```python
from build123d import *

# Parameters (mm, degrees)
SKETCH_1_R          = 3
EXTRUDE_1_DEPTH     = 8
SKETCH_2_R          = 1.5
CUT_EXTRUDE_1_DEPTH = 8
SKETCH_3_R          = 5
SKETCH_3_R_2        = 1.511526568
EXTRUDE_2_DEPTH     = 4


with BuildPart() as part:
    # 草图1 → 凸台-拉伸1 (new body)
    with BuildSketch(Plane(origin=(0, 0, 0), x_dir=(1, 0, 0), z_dir=(0, 1, 0))):
        with Locations(Location((0, 0, 0), (0, 0, 270))):
            Circle(SKETCH_1_R)
    extrude(amount=EXTRUDE_1_DEPTH)

    # 草图2 → 切除-拉伸1 (cut)
    with BuildSketch(Plane(origin=(0, 8, 0), x_dir=(1, 0, 0), z_dir=(0, 1, 0))):
        with Locations(Location((0, 0, 0), (0, 0, 270))):
            Circle(SKETCH_2_R)
    extrude(amount=-CUT_EXTRUDE_1_DEPTH, mode=Mode.SUBTRACT)

    # 草图3 → 凸台-拉伸2 (add)
    with BuildSketch(Plane.XZ):
        with Locations(Location((0, 0, 0), (0, 0, 270))):
            Circle(SKETCH_3_R)
        Circle(SKETCH_3_R_2, mode=Mode.SUBTRACT)
    extrude(amount=-EXTRUDE_2_DEPTH)


solid = part.part
```
The listing builds one solid part. Answer for the finished solid, in the listing's coordinates (mm). A direction names the side the tool comes from. Coordinates: 2 decimals unless noted, no trailing zeros. Loops run counter-clockwise (first coordinate to the right, second up) from the corner with the lowest first, then second, coordinate; pieces in that order, holes last. Notation, with made-up numbers: M 53,65 L 102,65 A20 ccw 102,80 Z; hole C -32,60 d4. An arc over 180 degrees is marked long. Answer as CSV lines item,"result". Start each with the question number.
(1) The mould has two halves that part along Z. Classify faces 3 (the flat face through (-1.3, 8, 1.3)), 4 (the cylindrical face through (0.9, 5.97, 2.86)), 5 (the cylindrical face through (0.45, 4.06, 1.43)): pulls with the +Z half, pulls with the -Z half, needs draft (parallel to the pull), parting line crosses it, or undercut.
(2) The part is cut by section D-D (z = -2.25). Give the vertices of the cut face in (x, y).
(3) The part is cut by section A-A (x = 0). Give the vertices of the cut face in (y, z).
(4) The part is cut by section B-B (z = 0). Give the vertices of the cut face in (x, y).
(5) Find the intervals of material crossed by L1, parallel to X at y = 0.75, z = 0; L2, parallel to Y at x = 1.25, z = 3; L3, parallel to Z at x = -1, y = 1.5, in increasing order. Write a range as [from, to].
(6) The part is cut by section C-C (y = 3.25). Give the vertices of the cut face in (x, z).
(7) Given pin 1 (1 mm diameter, centred on x = -2.5, y = 5, fed in from +Z); pin 2 (1.5 mm diameter, centred on y = 2, z = -1.5, fed in from +X), each flat-ended and moving along its own axis, determine where each tip first touches the part or whether it passes through.
(8) For faces 1 (the flat face through (-3.3, 4, 0.1)), 2 (the flat face through (1.2, 0, 1.2)), determine the directions among +Z, -Z, +X, -X, +Y, -Y from which every point of the face is accessible in a straight line to the end or side of a thin tool.
Determined:
1,face 3,"needs draft"
1,face 4,"parting line crosses it"
1,face 5,"undercut"
2,outline,"M -4.47,0 L 4.47,0 L 4.47,4 L 1.98,4 L 1.98,8 L -1.98,8 L -1.98,4 L -4.47,4 Z"
3,outline,"M 0,-5 L 4,-5 L 4,-3 L 8,-3 L 8,-1.5 L 0,-1.5 Z; M 0,1.5 L 8,1.5 L 8,3 L 4,3 L 4,5 L 0,5 Z"
4,outline,"M -5,0 L -1.5,0 L -1.5,8 L -3,8 L -3,4 L -5,4 Z; M 1.5,0 L 5,0 L 5,4 L 3,4 L 3,8 L 1.5,8 Z"
5,L1,"[-5, -1.5], [1.5, 5]"
5,L2,"[0, 4]"
5,L3,"[-4.9, -1.12], [1.12, 4.9]"
6,outline,"C 0,0 d10; hole C 0,0 d3"
7,pin 1,"z = 2.24"
7,pin 2,"x = 4.94"
8,face 1,"+Y"
8,face 2,"+Z, -Z, +X, -X, -Y"
